from build123d import *

# Parameters (mm, degrees)
SKETCH1_R           = 1
BOSS_EXTRUDE1_DEPTH = 1.55
SKETCH2_W           = 2.65
SKETCH2_H           = 2.65
BOSS_EXTRUDE2_DEPTH = 1
SKETCH3_W           = 12
SKETCH3_H           = 1
BOSS_EXTRUDE3_DEPTH = 1.3


with BuildPart() as part:
    # Sketch1 → Boss-Extrude1 (new body)
    with BuildSketch(Plane.XY):
        with BuildLine():
            Line((11.21, 14), (14.585786438, 14))
            Line((14.585786438, 14), (16, 12.585786438))
            Line((16, 12.585786438), (16, 0))
            Line((16, 0), (0, 0))
            Line((0, 0), (0, 12.585786438))
            Line((0, 12.585786438), (1.414213562, 14))
            Line((1.414213562, 14), (4.79, 14))
            ThreePointArc((4.79, 14), (5.355685425, 14.234314575), (5.59, 14.8))
            Line((5.59, 14.8), (5.59, 18.84))
            Line((5.59, 18.84), (10.41, 18.84))
            Line((10.41, 18.84), (10.41, 14.8))
            ThreePointArc((10.41, 14.8), (10.644314575, 14.234314575), (11.21, 14))
        make_face()
        with Locations(Location((2.575, 11.7, 0), (0, 0, 180))):
            Circle(SKETCH1_R, mode=Mode.SUBTRACT)
        with Locations(Location((13.425, 11.7, 0), (0, 0, 180))):
            Circle(SKETCH1_R, mode=Mode.SUBTRACT)
    extrude(amount=BOSS_EXTRUDE1_DEPTH)

    # Sketch2 → Boss-Extrude2 (add)
    with BuildSketch(Plane.XY.offset(1.55)):
        with Locations((8, 16.965)):
            Rectangle(SKETCH2_W, SKETCH2_H)
    extrude(amount=BOSS_EXTRUDE2_DEPTH)

    # Sketch3 → Boss-Extrude3 (add)
    with BuildSketch(Plane.XY.offset(1.55)):
        with Locations((8, 1.5)):
            Rectangle(SKETCH3_W, SKETCH3_H)
    extrude(amount=BOSS_EXTRUDE3_DEPTH)


solid = part.part
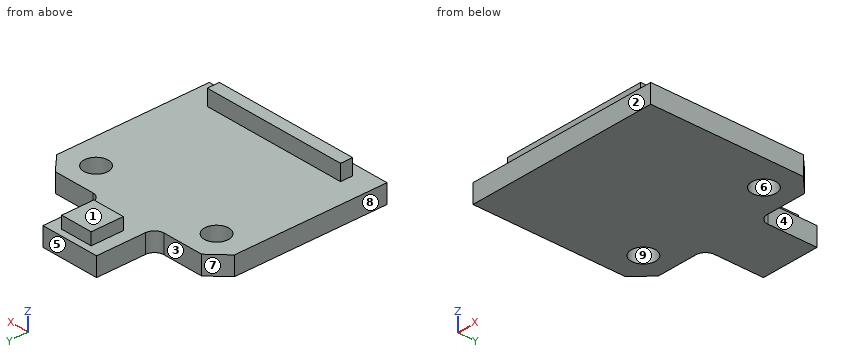
Could you check a few things on this model? Use its own coordinates, in mm. Face numbers are marked on the shaded views. A direction names the side the tool comes from. Round coordinates to 2 decimals unless told otherwise and drop trailing zeros. Order: outer loops, then holes, each group sorted by start corner. A loop starts at its lowest first (then second) coordinate and runs counter-clockwise, first axis right, second up.
Q1. Imagine slicing it at B-B, the plane y = 11.7. List the corners of the cut face in (x, z) for me (3 decimals), then the cut area to 3 significant figures.
Geometry says:
outline: (0, 0) - (1.575, 0) - (1.575, 1.55) - (0, 1.55) - close; (3.575, 0) - (12.425, 0) - (12.425, 1.55) - (3.575, 1.55) - close; (14.425, 0) - (16, 0) - (16, 1.55) - (14.425, 1.55) - close
area: 18.6 mm2
Q2. Imagine slicing it at C-C, the plane z = 0.2. List the corners of the cut face in (x, y) for me (3 decimals), then the cut area to 3 significant figures.
Geometry says:
outline: (0, 0) - (16, 0) - (16, 12.586) - (14.586, 14) - (11.21, 14) arc R0.8 cw to (10.41, 14.8) - (10.41, 18.84) - (5.59, 18.84) - (5.59, 14.8) arc R0.8 cw to (4.79, 14) - (1.414, 14) - (0, 12.586) - close; hole circle Ø2 at (2.575, 11.7); hole circle Ø2 at (13.425, 11.7)
area: 239 mm2
Q3. Thinking about a two-plate mould opening in Y: for the marked faces 6, 7, 8 and 9, which applies, released by +Y, released by -Y, zero draft, split by the parting line, or undercut?
Geometry says:
face 6: undercut
face 7: released by +Y
face 8: zero draft
face 9: undercut
Q4. Imagine slicing it at A-A, the plane z = 2. List the corners of the cut face in (x, y) for me (3 decimals), then the cut area to 3 significant figures.
Geometry says:
outline: (2, 1) - (14, 1) - (14, 2) - (2, 2) - close; (6.675, 15.64) - (9.325, 15.64) - (9.325, 18.29) - (6.675, 18.29) - close
area: 19.0 mm2
Q5. Which directions (+Z, -Z, +X, -X, +Y, -Y) give clear straight access to the entire face, cutting with the end or side of a thin tool? Please do the marked faces 1, 2, 3, 4 and 5.
Geometry says:
face 1: +Z, +X, -X, +Y
face 2: +Z, -Z, +X, -X, -Y
face 3: +Z, -Z, -X, +Y
face 4: +Z, -Z, +X, +Y
face 5: +Z, -Z, +X, -X, +Y
Q6. Please list where these lines run through material, in increasing order: probe 1 along X at (y, z) = (11.7, 0.5) (3 decimals); probe 2 along X at (y, z) = (12.25, 1.15); probe 3 along Y at (x, z) = (3.25, 2.05).
Geometry says:
probe 1: x = 0 to 1.575, 3.575 to 12.425, 14.425 to 16
probe 2: x = 0 to 1.74, 3.41 to 12.59, 14.26 to 16
probe 3: y = 1 to 2
Q7. Imagine slicing it at D-D, the plane x = 13.75. List the corners of the cut face in (y, z) for me, then the cut area to 3 significant figures.
Geometry says:
outline: (0, 0) - (10.75, 0) - (10.75, 1.55) - (2, 1.55) - (2, 2.85) - (1, 2.85) - (1, 1.55) - (0, 1.55) - close; (12.65, 0) - (14, 0) - (14, 1.55) - (12.65, 1.55) - close
area: 20.1 mm2
Q8. I'm going to push flat-ended pins straight in: P1, Ø4, axis at x = 8, y = 13, coming from the +Z side; P2, Ø1.2, axis at y = 17, z = 0.5, coming from the -X side; P3, Ø1.1, axis at y = 1.5, z = 2.5, coming from the -X side. Where does each tip first touch, or does it pass through?
Geometry says:
P1: stops at z = 1.55
P2: stops at x = 5.59
P3: stops at x = 2
